Autodesk Inventor part; units mm, degrees
ref_plane "YZ Plane" through (0, 0, 0) normal (1, 0, 0) x (0, 1, 0)
ref_plane "XZ Plane" through (0, 0, 0) normal (0, 1, 0) x (-1, 0, 0)
ref_plane "XY Plane" through (0, 0, 0) normal (0, 0, 1) x (1, 0, 0)
sketch "Sketch1" plane through (0, 0, 0) normal (0, 1, 0) x (-1, 0, 0)
  line L0 (3.175, 0) -> (98.425, 0)
  line L1 (101.6, 3.175) -> (101.6, 66.675)
  line L2 (98.425, 69.85) -> (3.175, 69.85)
  line L3 (0, 66.675) -> (0, 3.175)
  arc A0 (3.175, 69.85) -> (0, 66.675) centre (3.175, 66.675) ccw
  arc A1 (101.6, 66.675) -> (98.425, 69.85) centre (98.425, 66.675) ccw
  arc A2 (98.425, 0) -> (101.6, 3.175) centre (98.425, 3.175) ccw
  arc A3 (0, 3.175) -> (3.175, 0) centre (3.175, 3.175) ccw
  point P0 (0, 0)
  point P1 (101.6, 69.85)
  point P2 (101.6, 0)
  point P3 (0, 69.85)
  dimension "d0" = 101.6
  dimension "d1" = 69.85
  dimension "d13" = 3.175
extrude "Extrusion1" add sketch "Sketch1" along normal blind 3.175
sketch "Sketch2" plane through (0, 3.175, 0) normal (0, 1, 0) x (1, 0, 0)
  line L0 (-3.175, 0) -> (-98.425, 0)
  line L1 (-101.6, -3.175) -> (-101.6, -66.675)
  line L2 (0, -66.675) -> (0, -3.175)
  point P0 (0, 0)
  point P1 (-76.2, 0)
  point P2 (-76.2, -76.2)
  point P3 (-50.8, -38.1)
  dimension "d4" = 50.8
  dimension "d5" = 38.1
  dimension "d29" = 50.8
hole "Hole1" at (-50.8, 3.175, 38.1) direction (0, -1, 0) diameter 19.05 end through all
sketch "Sketch3" plane through (0, 3.175, 0) normal (0, 1, 0) x (1, 0, 0)
  line L0 (0, -66.675) -> (0, -3.175)
  line L1 (-101.6, -3.175) -> (-101.6, -66.675)
  circle A0 centre (-50.8, -38.1) radius 9.525
  point P0 (0, 0)
  point P1 (-85.725, -25.4)
  point P2 (-15.875, -25.4)
  point P3 (-9.525, -50.8)
  point P4 (-92.075, -50.8)
  dimension "d30" = 6.35
  dimension "d33" = 25.4
  dimension "d36" = 9.525
  dimension "d37" = 9.525
  dimension "d38" = 6.35
  dimension "d39" = 12.7
  dimension "d40" = 82.55
hole "Hole2" at (-85.725, 3.175, 25.4) at (-15.875, 3.175, 25.4) at (-9.525, 3.175, 50.8) at (-92.075, 3.175, 50.8) direction (0, -1, 0) diameter 6.35 end through all
properties part number "motorMount"
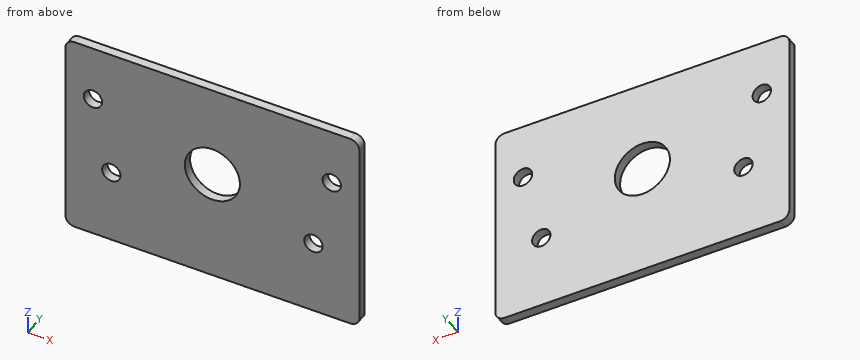
Could you check a few things on this model? Use its own coordinates, in mm. Coordinates: 2 decimals unless noted, no trailing zeros. Write each loop counter-clockwise with the first axis right and the second up, starting at its lowest first coordinate (ties: lowest second). Pieces come first, ordered by that corner, then holes. Notation, with made-up numbers: (42, 43.5) -> (81, 43.5) arc R22 cw to (81, 56.5) -> close; hole circle Ø1 at (54.5, -5.75). An arc over 180 degrees is marked (long way). Return JSON: item names as keys, results as strings.
(1) I need wall thicknesses on L1, parallel to X at y = 1.4, z = 25.4; L2, parallel to X at y = 1.95, z = 50.8; L3, parallel to Z at x = -50.8, y = 1.7 (3 decimals). Which ranges of each line are inside material? Lowest first, please.
Numbers:
{"L1": "x = -101.6 to -88.9, -82.55 to -19.05, -12.7 to 0", "L2": "x = -101.6 to -95.25, -88.9 to -12.7, -6.35 to 0", "L3": "z = 0 to 28.575, 47.625 to 69.85"}
(2) Imagine slicing it at B-B, the plane z = 25.4. Please give me the cut outline in (x, y) (3 decimals), then the cut area to 3 significant figures.
Numbers:
{"outline": "(-101.6, 0) -> (-88.9, 0) -> (-88.9, 3.175) -> (-101.6, 3.175) -> close; (-82.55, 0) -> (-19.05, 0) -> (-19.05, 3.175) -> (-82.55, 3.175) -> close; (-12.7, 0) -> (0, 0) -> (0, 3.175) -> (-12.7, 3.175) -> close", "area": "282 mm2"}
(3) Imagine slicing it at D-D, the plane z = 45. Please give me the cut outline in (x, y) (3 decimals), then the cut area to 3 significant figures.
Numbers:
{"outline": "(-101.6, 0) -> (-57.366, 0) -> (-57.366, 3.175) -> (-101.6, 3.175) -> close; (-44.234, 0) -> (0, 0) -> (0, 3.175) -> (-44.234, 3.175) -> close", "area": "281 mm2"}
(4) I'm going to push flat-ended pins straight in: pin 1 (8.5 mm diameter, centred on x = -85.725, z = 25.4, fed in from +Y) (3 decimals); pin 2 (5 mm diameter, centred on x = -15.875, z = 25.4, fed in from -Y). Where does each tip first touch, or does it pass through?
Numbers:
{"pin 1": "stops at y = 3.175", "pin 2": "passes through"}
(5) Imagine slicing it at A-A, the plane x = -50.8. Please give me the cut outline in (y, z) (3 decimals), then the cut area to 3 significant figures.
Numbers:
{"outline": "(0, 0) -> (3.175, 0) -> (3.175, 28.575) -> (0, 28.575) -> close; (0, 47.625) -> (3.175, 47.625) -> (3.175, 69.85) -> (0, 69.85) -> close", "area": "161 mm2"}
(6) Imagine slicing it at C-C, the plane y = 1.65. Please give me the cut outline in (x, z) (3 decimals), then the cut area to 3 significant figures.
Numbers:
{"outline": "(-101.6, 3.175) arc R3.175 ccw to (-98.425, 0) -> (-3.175, 0) arc R3.175 ccw to (0, 3.175) -> (0, 66.675) arc R3.175 ccw to (-3.175, 69.85) -> (-98.425, 69.85) arc R3.175 ccw to (-101.6, 66.675) -> close; hole circle Ø6.35 at (-92.075, 50.8); hole circle Ø6.35 at (-85.725, 25.4); hole circle Ø19.05 at (-50.8, 38.1); hole circle Ø6.35 at (-15.875, 25.4); hole circle Ø6.35 at (-9.525, 50.8)", "area": "6,680 mm2"}
